```python
from build123d import *

# Parameters (mm, degrees)
SKETCH1_W           = 89
SKETCH1_H           = 50
BOSS_EXTRUDE1_DEPTH = 1.5
SKETCH2_W           = 11.309347118
SKETCH2_H           = 21.514889616
SKETCH2_W_2         = 8.947956794
SKETCH2_H_2         = 4.853968999
SKETCH2_W_3         = 8.292015037
SKETCH2_H_3         = 10.757444808
SKETCH2_H_4         = 9.051996241
BOSS_EXTRUDE2_DEPTH = 15.5
SKETCH3_W           = 34.633694204
SKETCH3_H           = 21.121311428
BOSS_EXTRUDE3_DEPTH = 2


with BuildPart() as part:
    # Sketch1 → Boss-Extrude1 (new body)
    with BuildSketch(Plane(origin=(0, 0, 0), x_dir=(1, 0, 0), z_dir=(0, 1, 0))):
        Rectangle(SKETCH1_W, SKETCH1_H)
    extrude(amount=BOSS_EXTRUDE1_DEPTH)

    # Sketch2 → Boss-Extrude2 (add)
    with BuildSketch(Plane(origin=(0, 1.5, 0), x_dir=(1, 0, 0), z_dir=(0, 1, 0))):
        with Locations((-38.845326441, 8.199271957)):
            Rectangle(SKETCH2_W, SKETCH2_H)
        with Locations((-40.026021603, -12.725270077)):
            Rectangle(SKETCH2_W_2, SKETCH2_H_2)
        with Locations((40.353992482, 13.577994361)):
            Rectangle(SKETCH2_W_3, SKETCH2_H_3)
        with Locations((40.353992482, 1.96782527)):
            Rectangle(SKETCH2_W_3, SKETCH2_H_4)
    extrude(amount=BOSS_EXTRUDE2_DEPTH)

    # Sketch3 → Boss-Extrude3 (add)
    with BuildSketch(Plane(origin=(0, 1.5, 0), x_dir=(1, 0, 0), z_dir=(0, 1, 0))):
        Rectangle(SKETCH3_W, SKETCH3_H)
    extrude(amount=BOSS_EXTRUDE3_DEPTH)


solid = part.part
```
The listing builds one solid part. Answer for the finished solid, in the listing's coordinates (mm). A direction names the side the tool comes from. Coordinates: 2 decimals unless noted, no trailing zeros. Loops run counter-clockwise (first coordinate to the right, second up) from the corner with the lowest first, then second, coordinate; pieces in that order, holes last. Notation, with made-up numbers: (49, 28) -> (104, 28) arc R29 cw to (104, 57) -> close; hole circle Ø2 at (89.5, -7.5). An arc over 180 degrees is marked (long way). Return JSON: item names as keys, results as strings. Group by question number.
(1) A cutting plane is placed at A-A on y = 9.75. Write down the section's boundary in (x, z), and give its area (3 significant figures).
(2) Find the intervals of material crossed by probe 1 along Z at (x, y) = (41, 3.5); probe 2 along X at (y, z) = (6, -9); probe 3 along Y at (x, z) = (10.5, -3.5), in increasing order. Write a range as from..to.
(3) Determine the mould class of faces 6 (the flat face through (-17.317, 2, 0)), 7 (the flat face through (-1, 0, 0)), 8 (the flat face through (44.5, 8, -5)) for opening direction X: released by +X, released by -X, zero draft, split by the parting line, or undercut.
(4) A cutting plane is placed at D-D on x = -37. Write down the section's boundary in (y, z), and give its area (3 significant figures).
(5) A cutting plane is placed at C-C on z = 7. Write down the section's boundary in (x, y), and give its area (3 significant figures).
(6) Which of the six approach directions +Z, -Z, +X, -X, +Y, -Y give full straight-line access (tool end or side, diameter ignored) to faces 1 (the flat face through (0, 2, 10.561)), 2 (the flat face through (-40, 9, 15.152)), 3 (the flat face through (-40, 17, 13)), 4 (the flat face through (40, 9, -18.957)), 5 (the flat face through (-33.191, 9, -8))?
(7) Given pin 1 Ø10 at (x, z) = (-2, 19) entering from +Y; pin 2 Ø4.5 at (x, y) = (-39.5, 9.5) entering from +Z; pin 3 Ø2 at (x, y) = (-8.5, 3) entering from -Z; pin 4 Ø1.5 at (x, y) = (21.5, 3) entering from +Z, each flat-ended and moving along its own axis, determine where each tip first touches the part or whether it passes through.
(8) A cutting plane is placed at B-B on x = 3.5. Write down the section's boundary in (y, z).
The answers:
{
 "1": {"outline": "(-44.5, -18.96) -> (-33.19, -18.96) -> (-33.19, 2.56) -> (-44.5, 2.56) -> close; (-44.5, 10.3) -> (-35.55, 10.3) -> (-35.55, 15.15) -> (-44.5, 15.15) -> close; (36.21, -18.96) -> (44.5, -18.96) -> (44.5, -8.2) -> (36.21, -8.2) -> close; (36.21, -6.49) -> (44.5, -6.49) -> (44.5, 2.56) -> (36.21, 2.56) -> close", "area": "451 mm^2"},
 "2": {"probe 1": "z = -18.96..-8.2, -6.49..2.56", "probe 2": "x = -44.5..-33.19, 36.21..44.5", "probe 3": "y = 0..3.5"},
 "3": {"face 6": "undercut", "face 7": "zero draft", "face 8": "released by +X"},
 "4": {"outline": "(0, -25) -> (1.5, -25) -> (1.5, -18.96) -> (17, -18.96) -> (17, 2.56) -> (1.5, 2.56) -> (1.5, 10.3) -> (17, 10.3) -> (17, 15.15) -> (1.5, 15.15) -> (1.5, 25) -> (0, 25) -> close", "area": "484 mm^2"},
 "5": {"outline": "(-44.5, 0) -> (44.5, 0) -> (44.5, 1.5) -> (17.32, 1.5) -> (17.32, 3.5) -> (-17.32, 3.5) -> (-17.32, 1.5) -> (-44.5, 1.5) -> close", "area": "203 mm^2"},
 "6": {"face 1": "+Z, +X, +Y", "face 2": "+Z, +X, -X, +Y", "face 3": "+Z, -Z, +X, -X, +Y", "face 4": "-Z, +X, -X, +Y", "face 5": "+Z, -Z, +Y"},
 "7": {"pin 1": "stops at y = 1.5", "pin 2": "stops at z = 15.15", "pin 3": "stops at z = -10.56", "pin 4": "passes through"},
 "8": {"outline": "(0, -25) -> (1.5, -25) -> (1.5, -10.56) -> (3.5, -10.56) -> (3.5, 10.56) -> (1.5, 10.56) -> (1.5, 25) -> (0, 25) -> close"}
}
